Autodesk Inventor part; units mm, degrees
ref_plane "YZ Plane" through (0, 0, 0) normal (1, 0, 0) x (0, 1, 0)
ref_plane "XZ Plane" through (0, 0, 0) normal (0, 1, 0) x (-1, 0, 0)
ref_plane "XY Plane" through (0, 0, 0) normal (0, 0, 1) x (1, 0, 0)
sketch "Sketch1" plane through (0, 0, 0) normal (0, 0, 1) x (1, 0, 0)
  line L0 (-50, 70) -> (50, 70)
  line L1 (50, 0) -> (-50, 0)
  line L2 (0, 0) -> (0, 70) construction
  circle A0 centre (-17.5, 62) radius 1.6
  circle A1 centre (17.5, 62) radius 1.6
  arc A2 (-50, 70) -> (-53, 67) centre (-50, 67) ccw
  arc A3 (-53, 3) -> (-50, 0) centre (-50, 3) ccw
  arc A4 (53, 67) -> (50, 70) centre (50, 67) ccw
  arc A5 (50, 0) -> (53, 3) centre (50, 3) ccw
  line L3 (53, 67) -> (53, 3)
  line L4 (53, 20) -> (53, 3)
  line L5 (-53, 67) -> (-53, 3)
  line L6 (-53, 20) -> (-53, 3)
  point P0 (53, 45)
  point P1 (-53, 45)
  dimension "d11" = 70
  dimension "d20" = 3
  dimension "d22" = 3.2
  dimension "d23" = 8
  dimension "d24" = 35
  dimension "d31" = 106
extrude "Extrusion1" add sketch "Sketch1" along normal blind 3.175
sketch "Sketch2" plane through (0, 0, 3.175) normal (0, 0, 1) x (1, 0, 0)
  line L0 (-44, 57) -> (0, 57)
  line L1 (0, 0) -> (0, 57) construction
  line L2 (44, 57) -> (0, 57)
  line L3 (-50, -5) -> (50, -5)
  line L4 (-50, 0) -> (50, 0) construction
  arc A0 (50, 51) -> (44, 57) centre (44, 51) ccw
  arc A1 (-44, 57) -> (-50, 51) centre (-44, 51) ccw
  line L5 (50, 36) -> (46.8, 36)
  line L6 (46.8, 36) -> (46.8, 12)
  line L7 (46.8, 12) -> (50, 12)
  line L8 (-50, 36) -> (-46.8, 36)
  line L9 (-46.8, 36) -> (-46.8, 12)
  line L10 (-46.8, 12) -> (-50, 12)
  line L11 (50, -5) -> (50, 12)
  line L12 (50, 36) -> (50, 51)
  line L13 (-50, -5) -> (-50, 12)
  line L14 (-50, 36) -> (-50, 51)
  point P0 (47.5, 57)
  point P1 (-47.5, 57)
  dimension "d14" = 57
  dimension "d17" = 62
  dimension "d33" = 6
  dimension "d35" = 36
  dimension "d36" = 12
  dimension "d37" = 100
  dimension "d38" = 3.2
extrude "Extrusion2" cut sketch "Sketch2" against normal blind 6
properties part number "shovel"
Input: part model. Units: mm. Frame: model coordinates. A direction names the side the tool comes from. Round coordinates to 2 decimals unless told otherwise and drop trailing zeros. Order: outer loops, then holes, each group sorted by start corner. A loop starts at its lowest first (then second) coordinate and runs counter-clockwise, first axis right, second up. Notation, with made-up numbers: (-30.75, 22) - (26.25, 22) arc R16 ccw to (26.25, 34) - close; hole circle Ø2 at (61.25, 60). An arc over 180 degrees is marked (long way). Answer in a Markdown table with one row per item.
Item 1: Mould query, pull axis X, two halves, no side actions, for faces 1 (the flat face through (0, 58, 0)), 2 (the cylindrical face through (48.289, 55.196, 1.61)), 3 (the flat face through (53, 35, 2)). Classes: released by +X, released by -X, zero draft, split by the parting line, or undercut.
Model answer:
| item | result |
|---|---|
| face 1 | zero draft |
| face 2 | undercut |
| face 3 | released by +X |
Item 2: Reachability of faces 4 (the cylindrical face through (52.14, 0.9, 1.57)), 5 (the flat face through (48, 36, 2)), 6 (the flat face through (50, 6, 2)) from +Z, -Z, +X, -X, +Y, -Y: full face, straight path, thin tool, end or side. Return the list, or none.
Model answer:
| item | result |
|---|---|
| face 4 | +Z, -Z, +X, -Y |
| face 5 | +Z, -Z |
| face 6 | +Z, -Z, -Y |
Item 3: Section query C-C (x = -17.5). Return the cut outline in (y, z) (3 decimals).
Model answer:
| item | result |
|---|---|
| outline | (57, 0) - (60.4, 0) - (60.4, 3.175) - (57, 3.175) - close; (63.6, 0) - (70, 0) - (70, 3.175) - (63.6, 3.175) - close |
Item 4: Pin query (flat end, axial travel): pin 1 (1 mm diameter, centred on x = -48, z = 2, fed in from -Y). Return the tip coordinate at first contact, or that it passes through.
Model answer:
| item | result |
|---|---|
| pin 1 | stops at y = 12 |
Item 5: Section query D-D (x = 13.5). Return the cut outline in (y, z) (3 decimals).
Model answer:
| item | result |
|---|---|
| outline | (57, 0) - (70, 0) - (70, 3.175) - (57, 3.175) - close |
Item 6: Section query B-B (y = 62). Return the cut outline in (x, z) (3 decimals).
Model answer:
| item | result |
|---|---|
| outline | (-53, 0) - (-19.1, 0) - (-19.1, 3.175) - (-53, 3.175) - close; (-15.9, 0) - (15.9, 0) - (15.9, 3.175) - (-15.9, 3.175) - close; (19.1, 0) - (53, 0) - (53, 3.175) - (19.1, 3.175) - close |
Item 7: Line query: line 1 (X direction, y = 23, z = 2.9); line 2 (Y direction, x = -17.5, z = 1.85); line 3 (X direction, y = 48, z = 0.8). Output: solid intervals per line, ascending.
Model answer:
| item | result |
|---|---|
| line 1 | x = -53 to -46.8, 46.8 to 53 |
| line 2 | y = 57 to 60.4, 63.6 to 70 |
| line 3 | x = -53 to -50, 50 to 53 |
Item 8: Section query A-A (z = 1.8). Return the cut outline in (x, y).
Model answer:
| item | result |
|---|---|
| outline | (-53, 3) arc R3 ccw to (-50, 0) - (-50, 12) - (-46.8, 12) - (-46.8, 36) - (-50, 36) - (-50, 51) arc R6 cw to (-44, 57) - (44, 57) arc R6 cw to (50, 51) - (50, 36) - (46.8, 36) - (46.8, 12) - (50, 12) - (50, 0) arc R3 ccw to (53, 3) - (53, 67) arc R3 ccw to (50, 70) - (-50, 70) arc R3 ccw to (-53, 67) - close; hole circle Ø3.2 at (-17.5, 62); hole circle Ø3.2 at (17.5, 62) |
